Source: three-view drawing plus pictorial views. Frame: mm from the lowest corner of the part. A direction names the side the tool comes from. Round coordinates to 2 decimals unless told otherwise and drop trailing zeros. Answer in a Markdown table with one row per item. Add a question column.
Q1. Mould query, pull axis X, two halves, no side actions, for the marked faces 3, 4, 5 and 6. Classes: pulls with the +X half, pulls with the -X half, needs draft (parallel to the pull), parting line crosses it, or undercut.
Q2. Ray query, L1, parallel to Z at x = 123, y = 16.75 (1 decimal); L2, parallel to Z at x = 15, y = 9.5 (1 decimal); L3, parallel to Z at x = 21, y = 9.5 (1 decimal). Return the intervals inside material, ascending. Write a range as from..to.
Q3. Reachability of the marked faces 1 and 2 from +Z, -Z, +X, -X, +Y, -Y: full face, straight path, thin tool, end or side. Return the list, or none.
Q4. Section A-A, the plane x = 79.5. Give the number of separate pieces and of enclosed holes in the cut face, and give its area (3 significant figures).
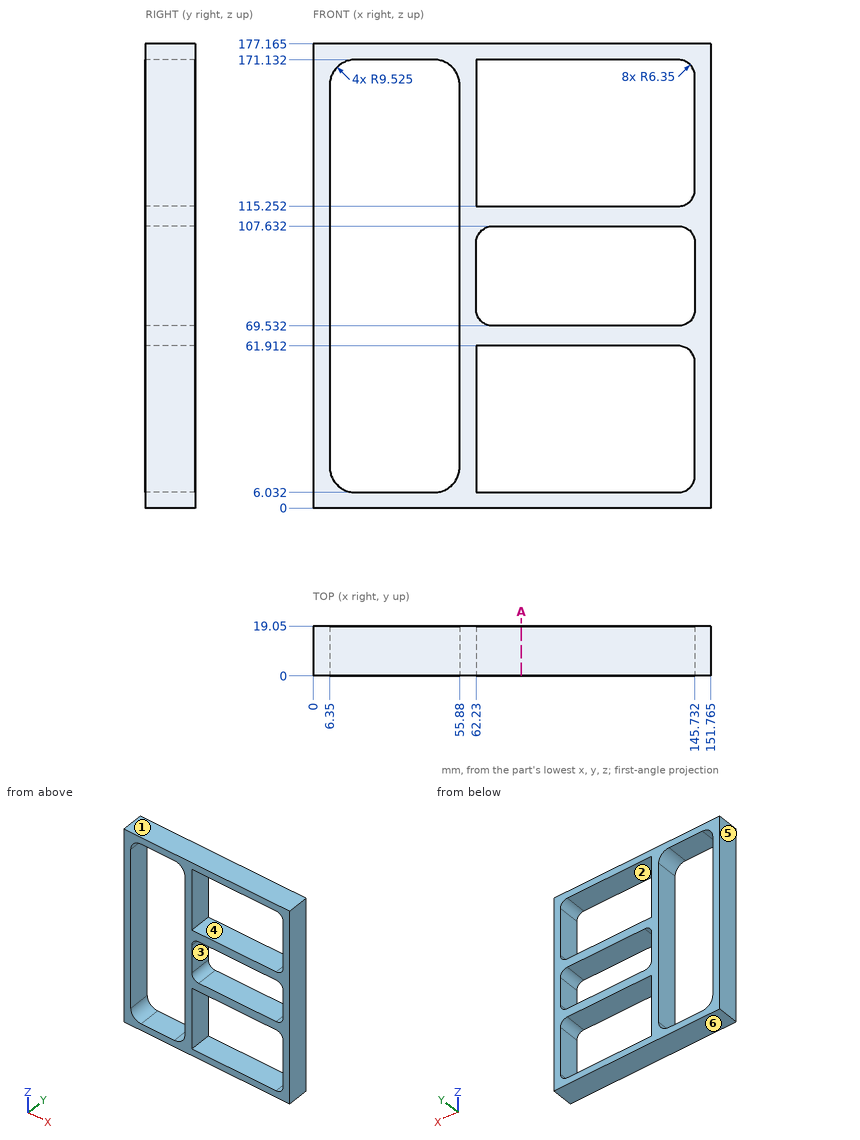
Answer block:
| question | item | result |
|---|---|---|
| 1 | face 3 | undercut |
| 1 | face 4 | undercut |
| 1 | face 5 | pulls with the -X half |
| 1 | face 6 | needs draft |
| 2 | L1 | 0..6, 61.9..69.5, 107.6..115.3, 171.1..177.2 |
| 2 | L2 | 0..6.1, 171.1..177.2 |
| 2 | L3 | 0..6, 171.1..177.2 |
| 3 | face 1 | +Z, +X, -X, +Y, -Y |
| 3 | face 2 | +Y, -Y |
| 4 | separate pieces | 4 |
| 4 | enclosed holes | 0 |
| 4 | area | 520 mm^2 |
